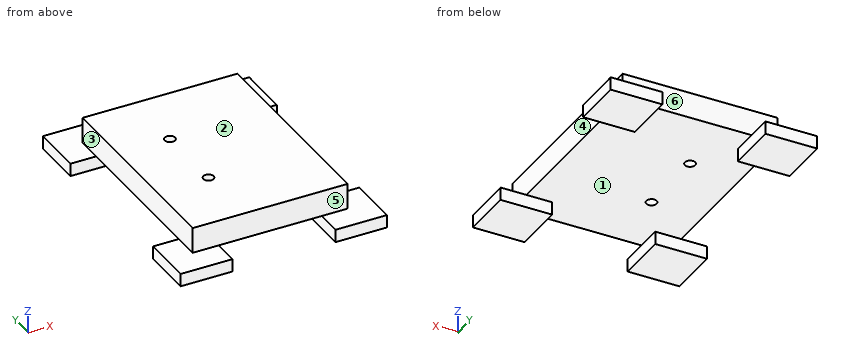
```python
from build123d import *

# Parameters (mm, degrees)
F0_W     = 38.1
F0_H     = 50.8
F1_DEPTH = 6.35
F2_W     = 12.7
F2_H     = 12.7
F3_DEPTH = 3.175
F4_R     = 1.2827
F5_DEPTH = 25.4


with BuildPart() as f1:
    # F0 (on Top) → F1 (new body)
    with BuildSketch(Plane.XY):
        with Locations((19.05, 25.4)):
            Rectangle(F0_W, F0_H)
    extrude(amount=F1_DEPTH)

    # F2 (on face) → F3 (join)
    with BuildSketch(Plane(origin=(0, 0, 0), x_dir=(1, 0, 0), z_dir=(0, 0, -1))):
        Rectangle(F2_W, F2_H)
        with Locations((38.1, 0)):
            Rectangle(F2_W, F2_H)
        with Locations((0, -50.8)):
            Rectangle(F2_W, F2_H)
        with Locations((38.1, -50.8)):
            Rectangle(F2_W, F2_H)
    extrude(amount=F3_DEPTH)

    # F4 (on face) → F5 (cut)
    with BuildSketch(Plane(origin=(0, 0, 0), x_dir=(1, 0, 0), z_dir=(0, 0, -1))):
        with Locations((12.7, -16.51)):
            Circle(F4_R)
        with Locations((12.7, -34.29)):
            Circle(F4_R)
    extrude(amount=-F5_DEPTH, mode=Mode.SUBTRACT)


solid = f1.part
```
Geometry check sheet. Reference: the model listing, model coordinates, mm. Face numbers are marked on the shaded views. A direction names the side the tool comes from. Coordinates: 2 decimals unless noted, no trailing zeros. Loops run counter-clockwise (first coordinate to the right, second up) from the corner with the lowest first, then second, coordinate; pieces in that order, holes last. Notation, with made-up numbers: (-28, 4) -> (-20, 4) arc R26 ccw to (-20, 42) -> close; hole circle Ø5 at (-9, 60.25). An arc over 180 degrees is marked (long way). Put each result on its own line as item: value.
1) Cross-section at B-B on y = 34.29. Record the boundary of the cut face in (x, z).
Result set:
outline: (0, 0) -> (11.42, 0) -> (11.42, 6.35) -> (0, 6.35) -> close; (13.98, 0) -> (38.1, 0) -> (38.1, 6.35) -> (13.98, 6.35) -> close
2) Gauge pin test, flat ends, axial feed: pin 1 Ø5 at (x, z) = (28, 2) entering from +Y; pin 2 Ø2 at (y, z) = (46, 5) entering from -X; pin 3 Ø4 at (x, y) = (12.7, 34.29) entering from -Z. Record the tip position at first contact, or that the pin passes through.
Result set:
pin 1: stops at y = 50.8
pin 2: stops at x = 0
pin 3: stops at z = 0
3) Thickness scan on line 1 (Y direction, x = 12.7, z = 1.75); line 2 (X direction, y = 16.51, z = 2); line 3 (X direction, y = 28.5, z = 3). Record the ranges inside material, lowest first.
Result set:
line 1: y = 0 to 15.23, 17.79 to 33.01, 35.57 to 50.8
line 2: x = 0 to 11.42, 13.98 to 38.1
line 3: x = 0 to 38.1
4) Release check for a two-part mould opening along X. For the marked faces 1, 2 and 3 record: released by +X, released by -X, zero draft, split by the parting line, or undercut.
Result set:
face 1: undercut
face 2: zero draft
face 3: released by -X
5) Cross-section at D-D on z = 4.5. Record the boundary of the cut face in (x, y).
Result set:
outline: (0, 0) -> (38.1, 0) -> (38.1, 50.8) -> (0, 50.8) -> close; hole circle Ø2.57 at (12.7, 16.51); hole circle Ø2.57 at (12.7, 34.29)
6) Cross-section at A-A on z = -1.25. Record the boundary of the cut face in (x, y).
Result set:
outline: (-6.35, -6.35) -> (6.35, -6.35) -> (6.35, 6.35) -> (-6.35, 6.35) -> close; (-6.35, 44.45) -> (6.35, 44.45) -> (6.35, 57.15) -> (-6.35, 57.15) -> close; (31.75, -6.35) -> (44.45, -6.35) -> (44.45, 6.35) -> (31.75, 6.35) -> close; (31.75, 44.45) -> (44.45, 44.45) -> (44.45, 57.15) -> (31.75, 57.15) -> close
7) Cross-section at C-C on x = 35.5. Record the boundary of the cut face in (y, z) (3 decimals).
Result set:
outline: (-6.35, -3.175) -> (6.35, -3.175) -> (6.35, 0) -> (44.45, 0) -> (44.45, -3.175) -> (57.15, -3.175) -> (57.15, 0) -> (50.8, 0) -> (50.8, 6.35) -> (0, 6.35) -> (0, 0) -> (-6.35, 0) -> close
8) Tool access check on the marked faces 4, 5 and 6. Record the directions out of +Z, -Z, +X, -X, +Y, -Y that give a thin tool (end or side, any length) a straight path to the whole face; none if there is none.
Result set:
face 4: +Z, +X, +Y, -Y
face 5: +Z, +X, -X, -Y
face 6: +Z, +X, -X, +Y
